Source: three-view drawing plus pictorial views. Frame: mm from the lowest corner of the part. Coordinates: 2 decimals unless noted, no trailing zeros. Write each loop counter-clockwise with the first axis right and the second up, starting at its lowest first coordinate (ties: lowest second). Pieces come first, ordered by that corner, then holes. Notation, with made-up numbers: (-36, 15.5) - (8, 15.5) arc R34 cw to (8, 52.5) - close; hole circle Ø8 at (21.25, 15.25). An arc over 180 degrees is marked (long way). One line per item, written item: value.
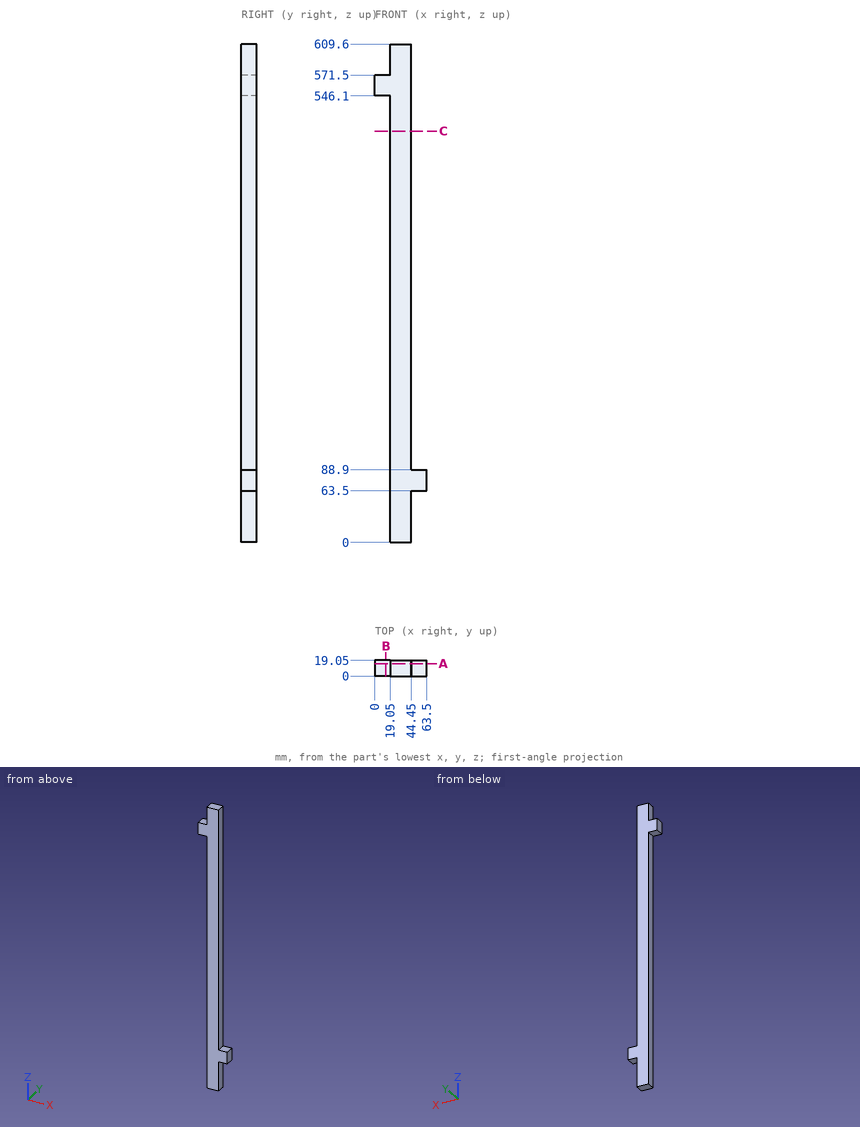
1) Section query C-C on z = 503. Output: boundary loops of the cut face in (x, y), then the cut area to 3 significant figures.
Values found:
outline: (19.05, 0) - (44.45, 0) - (44.45, 19.05) - (19.05, 19.05) - close
area: 484 mm2
2) Section query A-A on y = 15.25. Output: boundary loops of the cut face in (x, z), then the cut area to 3 significant figures.
Values found:
outline: (0, 546.1) - (19.05, 546.1) - (19.05, 0) - (44.45, 0) - (44.45, 63.5) - (63.5, 63.5) - (63.5, 88.9) - (44.45, 88.9) - (44.45, 609.6) - (19.05, 609.6) - (19.05, 571.5) - (0, 571.5) - close
area: 16,500 mm2
3) Material intervals for line 1 (X direction, y = 4.5, z = 557); line 2 (X direction, y = 3.75, z = 528); line 3 (Z direction, x = 12.5, y = 5.5), sorted ascending.
Values found:
line 1: 0 to 44.45
line 2: 19.05 to 44.45
line 3: 546.1 to 571.5
4) Section query B-B on x = 13.5. Output: boundary loops of the cut face in (y, z).
Values found:
outline: (0, 546.1) - (19.05, 546.1) - (19.05, 571.5) - (0, 571.5) - close
5) Contact query for flat-ended pins moving along their axis: P1, Ø1.5, axis at y = 6, z = 316, coming from the +X side; P2, Ø5, axis at x = 21, y = 8.5, coming from the -Z side; P3, Ø10, axis at x = 13.5, z = 261.5, coming from the +Y side; P4, Ø5, axis at x = 8.5, y = 3, coming from the +Z side. Output: stop coordinate, or through.
Values found:
P1: x = 44.45
P2: z = 0
P3: through
P4: z = 571.5
